Source: CAD feature listing. Evaluate the final solid. Frame: model axes, mm. A direction names the side the tool comes from. Give positions to 0.01 mm unless a question says otherwise; leave off trailing zeros. Loops run counter-clockwise (first coordinate to the right, second up) from the corner with the lowest first, then second, coordinate; pieces in that order, holes last.
from build123d import *

# Parameters (mm, degrees)
BOSS_EXTRUDE1_DEPTH  = 1
BOSS_EXTRUDE2_DEPTH  = 2
BOSS_EXTRUDE3_DEPTH  = 3
BOSS_EXTRUDE4_DEPTH  = 5
BOSS_EXTRUDE5_DEPTH  = 8
BOSS_EXTRUDE6_DEPTH  = 13
BOSS_EXTRUDE7_DEPTH  = 21
BOSS_EXTRUDE8_DEPTH  = 34
BOSS_EXTRUDE9_DEPTH  = 55
BOSS_EXTRUDE10_DEPTH = 178


with BuildPart() as part:
    # Sketch1 → Boss-Extrude1 (new body)
    with BuildSketch(Plane(origin=(0, 0, 0), x_dir=(1, 0, 0), z_dir=(0, 1, 0))):
        Polygon((1, 0), (0, 0), (0, -0.997190903), (2.001284941, -0.997190903), (2.001284941, 1), (1, 1), align=None)
    extrude(amount=BOSS_EXTRUDE1_DEPTH)

    # Sketch1_3 → Boss-Extrude2 (add)
    with BuildSketch(Plane(origin=(0, 0, 0), x_dir=(1, 0, 0), z_dir=(0, 1, 0))):
        Polygon((1, 1), (2.001284941, 1), (2.001284941, 2.997699814), (-1, 2.997699814), (-1, 1), align=None)
    extrude(amount=BOSS_EXTRUDE2_DEPTH)

    # Sketch1_4 → Boss-Extrude3 (add)
    with BuildSketch(Plane(origin=(0, 0, 0), x_dir=(1, 0, 0), z_dir=(0, 1, 0))):
        Polygon((-1, 2.997699814), (-3.999741098, 2.997699814), (-3.999741098, -2), (-1, -2), (-1, 1), align=None)
    extrude(amount=BOSS_EXTRUDE3_DEPTH)

    # Sketch1_5 → Boss-Extrude4 (add)
    with BuildSketch(Plane(origin=(0, 0, 0), x_dir=(1, 0, 0), z_dir=(0, 1, 0))):
        Polygon((4, -2), (4, -6.996932288), (-3.999741098, -6.996932288), (-3.999741098, -2), (-1, -2), align=None)
    extrude(amount=BOSS_EXTRUDE4_DEPTH)

    # Sketch1_6 → Boss-Extrude5 (add)
    with BuildSketch(Plane(origin=(0, 0, 0), x_dir=(1, 0, 0), z_dir=(0, 1, 0))):
        Polygon((4, -6.996932288), (12.003242926, -6.996932288), (12.003242926, 6), (4, 6), (4, -2), align=None)
    extrude(amount=BOSS_EXTRUDE5_DEPTH)

    # Sketch1_7 → Boss-Extrude6 (add)
    with BuildSketch(Plane(origin=(0, 0, 0), x_dir=(1, 0, 0), z_dir=(0, 1, 0))):
        Polygon((-9, 6), (-9, 18.995575243), (12.003242926, 18.995575243), (12.003242926, 6), (4, 6), align=None)
    extrude(amount=BOSS_EXTRUDE6_DEPTH)

    # Sketch1_8 → Boss-Extrude7 (add)
    with BuildSketch(Plane(origin=(0, 0, 0), x_dir=(1, 0, 0), z_dir=(0, 1, 0))):
        Polygon((-9, 18.995575243), (-30.000063684, 18.995575243), (-30.000063684, -15), (-9, -15), (-9, 6), align=None)
    extrude(amount=BOSS_EXTRUDE7_DEPTH)

    # Sketch1_9 → Boss-Extrude8 (add)
    with BuildSketch(Plane(origin=(0, 0, 0), x_dir=(1, 0, 0), z_dir=(0, 1, 0))):
        Polygon((25, -15), (25, -49.004916202), (-30.000063684, -49.004916202), (-30.000063684, -15), (-9, -15), align=None)
    extrude(amount=BOSS_EXTRUDE8_DEPTH)

    # Sketch1_10 → Boss-Extrude9 (add)
    with BuildSketch(Plane(origin=(0, 0, 0), x_dir=(1, 0, 0), z_dir=(0, 1, 0))):
        Polygon((25, -49.004916202), (79.998803233, -49.004916202), (79.998803233, 40), (25, 40), (25, -15), align=None)
    extrude(amount=BOSS_EXTRUDE9_DEPTH)

    # Sketch1_12 → Boss-Extrude10 (add)
    with BuildSketch(Plane(origin=(0, 0, 0), x_dir=(1, 0, 0), z_dir=(0, 1, 0))):
        Polygon((-64, 40), (-64, 128.996056825), (79.998803233, 128.996056825), (79.998803233, 40), (25, 40), align=None)
    extrude(amount=BOSS_EXTRUDE10_DEPTH)


solid = part.part
1) Cut plane A-A (x = 20.5). Return loops of the section in (y, z), and give its area (3 significant figures).
Checks:
outline: (0, -129) - (178, -129) - (178, -40) - (0, -40) - close; (0, 15) - (34, 15) - (34, 49) - (0, 49) - close
area: 17,000 mm2
2) Contact query for flat-ended pins moving along their axis: P1, Ø5.5, axis at x = 0.5, z = 3.5, coming from the +Y side; P2, Ø1.5, axis at x = 20.5, y = 132.5, coming from the +Z side; P3, Ø12, axis at x = -21.5, z = -29.5, coming from the +Y side; P4, Ø1.1, axis at y = 0.5, z = -0.5, coming from the -X side. Output: stop coordinate, or through.
Checks:
P1: stops at y = 5
P2: stops at z = -40
P3: passes through
P4: stops at x = -30
3) Cut plane B-B (y = 42). Return loops of the section in (x, z), and give its area (3 significant figures).
Checks:
outline: (-64, -129) - (80, -129) - (80, 49) - (25, 49) - (25, -40) - (-64, -40) - close
area: 17,700 mm2
4) Reachability of faces 4 (the flat face through (4, 17, 15)), 5 (the flat face through (-2, 34, 32)), 6 (the flat face through (-20, 21, -2)) from +Z, -Z, +X, -X, +Y, -Y: full face, straight path, thin tool, end or side. Return the list, or none.
Checks:
face 4: +Y
face 5: +Z, -X, +Y
face 6: -X, +Y
5) Cut plane C-C (x = 66.5). Return loops of the section in (y, z), and give its area (3 significant figures).
Checks:
outline: (0, -129) - (178, -129) - (178, -40) - (55, -40) - (55, 49) - (0, 49) - close
area: 20,700 mm2
6) Pull-direction query (Z, two-part tool) for faces 1 (the flat face through (7, 88, -128.996)), 2 (the flat face through (2, 13, -13)), 3 (the flat face through (9, 0, -41)); classes: released by +Z, released by -Z, zero draft, split by the parting line, or undercut.
Checks:
face 1: released by -Z
face 2: undercut
face 3: zero draft
7) Ray query, probe 1 along Z at (x, y) = (-56.5, 130); probe 2 along Y at (x, z) = (43.5, 17); probe 3 along X at (y, z) = (18, 21). Return the intervals inside material, ascending.
Checks:
probe 1: z = -129 to -40
probe 2: y = 0 to 55
probe 3: x = -30 to 80
8) Cut plane D-D (y = 66). Return loops of the section in (x, z).
Checks:
outline: (-64, -129) - (80, -129) - (80, -40) - (-64, -40) - close
